Source: three-view drawing plus pictorial views. Frame: mm from the lowest corner of the part. A direction names the side the tool comes from. Give positions to 0.01 mm unless a question says otherwise; leave off trailing zeros. Order: outer loops, then holes, each group sorted by start corner. A loop starts at its lowest first (then second) coordinate and runs counter-clockwise, first axis right, second up. Notation, with made-up numbers: M 21.25,34.5 L 39.25,34.5 A25 cw 39.25,66.5 Z; hole C 34.25,56.5 d8. An arc over 180 degrees is marked long. Use CSV: the item, a comma, the result in double quotes.
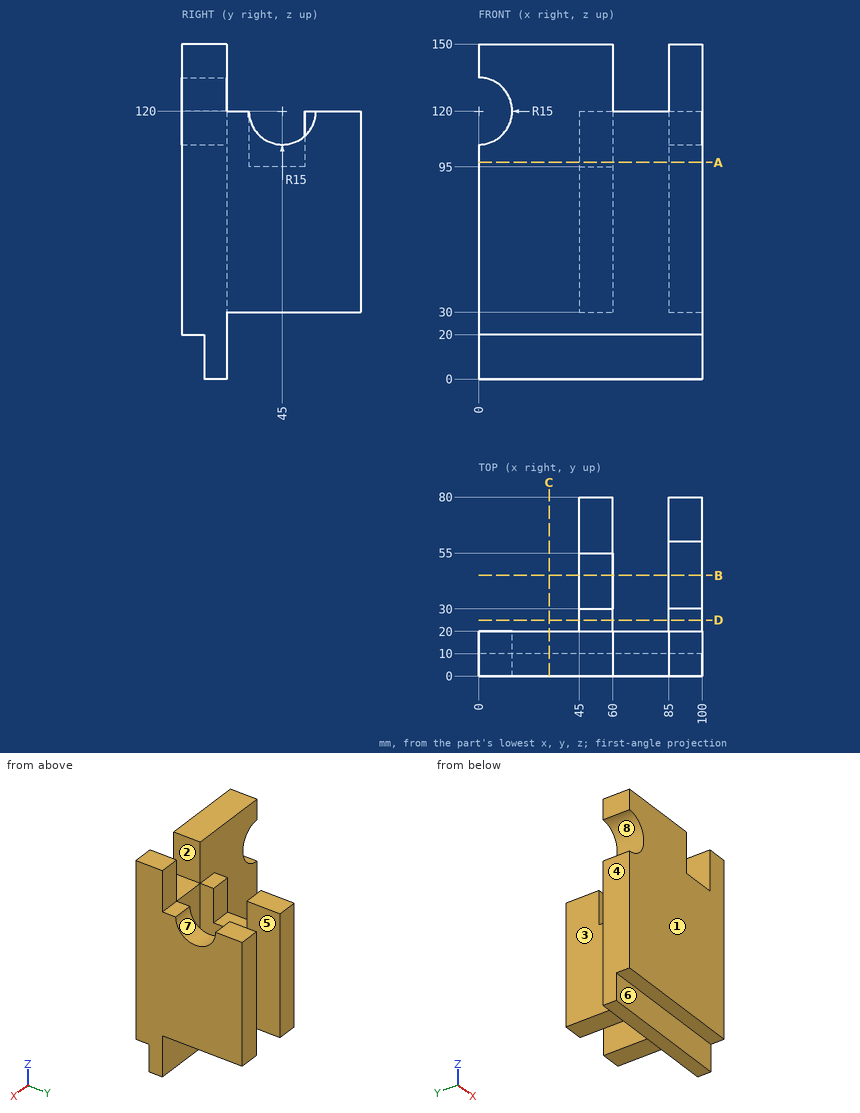
1. Pin query (flat end, axial travel): pin 1 Ø7.5 at (x, y) = (54, 40) entering from +Z; pin 2 Ø12 at (x, y) = (92, 57.5) entering from -Z; pin 3 Ø1 at (x, z) = (19.5, 95) entering from +Y. Return the tip coordinate at first contact, or that it passes through.
Answer:
pin 1,"z = 95"
pin 2,"z = 30"
pin 3,"y = 20"
2. Section D-D, the plane y = 25. Return the cut outline in (x, z), plus the area to 3 significant figures.
Answer:
outline,"M 45,30 L 60,30 L 60,120 L 45,120 Z; M 85,30 L 100,30 L 100,120 L 85,120 Z"
area,"2,700 mm2"
3. Section C-C, the plane x = 31.5. Return the cut outline in (y, z), plus the area to 3 significant figures.
Answer:
outline,"M 0,20 L 10,20 L 10,0 L 20,0 L 20,150 L 0,150 Z"
area,"2,800 mm2"
4. Line query: line 1 (X direction, y = 23, z = 110.5); line 2 (Z direction, x = 92, y = 75); line 3 (Y direction, x = 80.5, z = 55). Output: solid intervals per line, ascending.
Answer:
line 1,"45 to 60, 85 to 100"
line 2,"30 to 120"
line 3,"0 to 20"
5. Reachability of the marked faces 1, 2, 3, 4 and 5 from +Z, -Z, +X, -X, +Y, -Y: full face, straight path, thin tool, end or side. Return the list, or none.
Answer:
face 1,"+Z, -Z, +X, -X, -Y"
face 2,"+Z, +Y, -Y"
face 3,"+Z, -Z, -X, +Y"
face 4,"+Z, -Z, -X, +Y, -Y"
face 5,"+Z, -Z, +Y"
6. Pull-direction query (Z, two-part tool) for the marked faces 6, 7 and 8; classes: +Z half, -Z half, draft (parallel to the pull), parting line (faces both ways), or undercut.
Answer:
face 6,"draft"
face 7,"+Z half"
face 8,"undercut"
7. Section B-B, the plane y = 45. Return the cut outline in (x, z), plus the area to 3 significant figures.
Answer:
outline,"M 45,30 L 60,30 L 60,95 L 45,95 Z; M 85,30 L 100,30 L 100,105 L 85,105 Z"
area,"2,100 mm2"
8. Section A-A, the plane z = 97. Return the cut outline in (x, y), plus the area to 4 significant figures.
Answer:
outline,"M 0,0 L 100,0 L 100,80 L 85,80 L 85,20 L 60,20 L 60,30 L 45,30 L 45,20 L 0,20 Z; M 45,55 L 60,55 L 60,80 L 45,80 Z"
area,"3,425 mm2"
